from build123d import *

# Parameters (mm, degrees)
F0_R     = 3.9751
F1_DEPTH = 3.175
F2_W     = 34.925
F2_H     = 22.225
F2_R     = 4.7625
F3_DEPTH = 6.35
F4_R     = 5.08


with BuildPart() as f1:
    # F0 (on Top) → F1 (new body, symmetric)
    with BuildSketch(Plane.XY):
        Polygon((0, 19.05), (0, 0), (28.575, 0), (28.575, 31.75), (-34.925, 31.75), (-34.925, 19.05), align=None)
        with Locations((15.875, 12.7)):
            Circle(F0_R, mode=Mode.SUBTRACT)
    extrude(amount=F1_DEPTH, both=True)

    # F2 (on face) → F3 (join)
    with BuildSketch(Plane.XZ.offset(-19.05)):
        with Locations((-17.4625, 14.2875)):
            Rectangle(F2_W, F2_H)
        with Locations((-17.4625, 14.2875)):
            Circle(F2_R, mode=Mode.SUBTRACT)
    extrude(amount=-F3_DEPTH)

    # F4
    f4_edges = [f1.edges().sort_by_distance(p)[0] for p in [
        (-34.925, 22.225, 25.4),
        (0, 22.225, 25.4),
        (0, 0, 0),
        (28.575, 0, 0),
    ]]
    fillet(f4_edges, radius=F4_R)


solid = f1.part
Read the model definition and answer for the solid it produces. Units are mm, in the model's axes. A direction names the side the tool comes from. Coordinates: 2 decimals unless noted, no trailing zeros. Loops run counter-clockwise (first coordinate to the right, second up) from the corner with the lowest first, then second, coordinate; pieces in that order, holes last.
Q1. Each of these flat-tipped pins is pushed along its axis until it touches: pin 1 Ø5 at (y, z) = (9.5, -1) entering from -X; pin 2 Ø7 at (y, z) = (22, 11) entering from +X; pin 3 Ø8.5 at (x, z) = (-10, 11.5) entering from -Y; pin 4 Ø5 at (x, y) = (15.875, 12.7) entering from -Z. Where does it stop, or does it pass through?
Q2. The part is cut by section B-B on y = 24. Write down the section's boundary in (x, z) (1 decimal).
Q3. The part is cut by section C-C on z = 13. Write down the section's boundary in (x, y) (3 decimals).
Q4. The part is cut by section D-D on x = -7. Write down the section's boundary in (y, z) (3 decimals), and give its area (3 significant figures).
Q5. Consider probe 1 along Y at (x, z) = (-12.5, 23.25); probe 2 along Z at (x, y) = (23.5, 11) (3 decimals); probe 3 along Y at (x, z) = (-22, 1.5). Determine where each line is inside the solid, lowest interval first.
Q6. The mould has two halves that part along X. Classify faces 4 (the face through (3, 20, -3.175)), 5 (the face through (1.449, 1.528, 0.044)), 6 (the face through (15.01, 8.82, -0.04)): +X half, -X half, draft (parallel to the pull), parting line (faces both ways), or undercut.
Q7. The part is cut by section A-A on y = 12.7. Write down the section's boundary in (x, z) (3 decimals).
Q8. Which of the six approach directions +Z, -Z, +X, -X, +Y, -Y give full straight-line access (tool end or side, diameter ignored) to faces 1 (the face through (-22, 25.4, 17)), 2 (the face through (0, 12, 0)), 3 (the face through (0, 22, 12))?
Results below:
1. pin 1: stops at x = 0
1. pin 2: stops at x = 0
1. pin 3: stops at y = 19.05
1. pin 4: passes through
2. outline: (-34.9, -3.2) - (28.6, -3.2) - (28.6, 3.2) - (0, 3.2) - (0, 20.3) arc R5.1 ccw to (-5.1, 25.4) - (-29.8, 25.4) arc R5.1 ccw to (-34.9, 20.3) - close; hole circle Ø9.5 at (-17.5, 14.3)
3. outline: (-34.925, 19.05) - (-22.048, 19.05) - (-22.048, 25.4) - (-34.925, 25.4) - close; (-12.877, 19.05) - (0, 19.05) - (0, 25.4) - (-12.877, 25.4) - close
4. outline: (19.05, -3.175) - (31.75, -3.175) - (31.75, 3.175) - (25.4, 3.175) - (25.4, 25.4) - (19.05, 25.4) - close
4. area: 222 mm2
5. probe 1: y = 19.05 to 25.4
5. probe 2: z = -3.175 to 3.175
5. probe 3: y = 19.05 to 31.75
6. face 4: draft
6. face 5: -X half
6. face 6: undercut
7. outline: (0, -3.175) - (11.9, -3.175) - (11.9, 3.175) - (0, 3.175) - close; (19.85, -3.175) - (28.575, -3.175) - (28.575, 3.175) - (19.85, 3.175) - close
8. face 1: +Z, +X, -X, +Y
8. face 2: +Z, -Z, -X, -Y
8. face 3: +Z, +X, +Y, -Y
